For this review, take the finished solid that the model builds, in its own axes (mm). Round coordinates to 2 decimals unless told otherwise and drop trailing zeros. Answer in a Markdown table with one row per item. Add a question column.
from build123d import *

# Parameters (mm, degrees)
SKETCH1_W           = 52
SKETCH1_H           = 18
BOSS_EXTRUDE1_DEPTH = 6.55
FILLET1_R           = 2
FILLET2_R           = 1
SKETCH2_W           = 45
SKETCH2_H           = 14
CUT_EXTRUDE1_DEPTH  = 0.01
SKETCH3_W           = 14
SKETCH3_H           = 8
CUT_EXTRUDE2_DEPTH  = 0.01


with BuildPart() as part:
    # Sketch1 → Boss-Extrude1 (new, symmetric)
    with BuildSketch(Plane(origin=(0, 0, 0), x_dir=(1, 0, 0), z_dir=(0, 1, 0))):
        Rectangle(SKETCH1_W, SKETCH1_H)
    extrude(amount=BOSS_EXTRUDE1_DEPTH, both=True)

    # Fillet1
    fillet1_edges = [part.edges().sort_by_distance(p)[0] for p in [
        (-26, 6.55, 0),
        (26, 6.55, 0),
        (-26, -6.55, 0),
        (26, -6.55, 0),
    ]]
    fillet(fillet1_edges, radius=FILLET1_R)

    # Fillet2
    fillet2_edges = [part.edges().sort_by_distance(p)[0] for p in [
        (-26, 0, 9),
        (-26, 0, -9),
        (0, -6.55, 9),
        (26, 0, 9),
        (0, 6.55, 9),
        (25.414213562, 5.964213562, 9),
        (25.414213562, -5.964213562, 9),
        (-25.414213562, 5.964213562, 9),
        (-25.414213562, -5.964213562, 9),
        (0, -6.55, -9),
        (0, 6.55, -9),
        (26, 0, -9),
        (25.414213562, 5.964213562, -9),
        (25.414213562, -5.964213562, -9),
        (-25.414213562, 5.964213562, -9),
        (-25.414213562, -5.964213562, -9),
    ]]
    fillet(fillet2_edges, radius=FILLET2_R)

    # Sketch2 → Cut-Extrude1 (cut)
    with BuildSketch(Plane(origin=(0, 6.55, 0), x_dir=(1, 0, 0), z_dir=(0, 1, 0))):
        Rectangle(SKETCH2_W, SKETCH2_H)
    cut_extrude1 = extrude(amount=-CUT_EXTRUDE1_DEPTH, mode=Mode.SUBTRACT)

    # Sketch3 → Cut-Extrude2 (cut)
    with BuildSketch(Plane.ZY.offset(26)):
        Rectangle(SKETCH3_W, SKETCH3_H)
    cut_extrude2 = extrude(amount=-CUT_EXTRUDE2_DEPTH, mode=Mode.SUBTRACT)

    # Mirror3: Cut-Extrude1 across plane
    add(cut_extrude1.mirror(Plane.ZX), mode=Mode.SUBTRACT)

    # Mirror4: Cut-Extrude2 across plane
    add(cut_extrude2.mirror(Plane(origin=(0, 0, 0), x_dir=(0, 0, 1), z_dir=(1, 0, 0))), mode=Mode.SUBTRACT)


solid = part.part
Q1. Insertion check: pin 1 Ø1 at (x, z) = (13, 2) entering from -Y; pin 2 Ø3 at (y, z) = (-1, -3.5) entering from -X; pin 3 Ø1.5 at (x, z) = (-20.5, 2.5) entering from +Y. Each pin has a flat end and moves straight along its axis. Give the tip position at first contact, or say it passes through.
Q2. Draft analysis for pull direction Y (two halves, no side actions). For faces 1 (the face through (-25.43, 5.95, -0.11)), 2 (the face through (-0.1, -6.55, 7.7)), 3 (the face through (-26, -4.4, 0)), state which applies: released by +Y, released by -Y, zero draft, split by the parting line, or undercut.
Q3. To check wall thickness, follow probe 1 along X at (y, z) = (-4.75, 8); probe 2 along Y at (x, z) = (-22, -0.5); probe 3 along Y at (x, z) = (-18.5, -8.5). State the ranges of each line that lie inside material, in increasing order.
Answer sheet:
| question | item | result |
|---|---|---|
| 1 | pin 1 | stops at y = -6.54 |
| 1 | pin 2 | stops at x = -25.99 |
| 1 | pin 3 | stops at y = 6.54 |
| 2 | face 1 | released by +Y |
| 2 | face 2 | released by -Y |
| 2 | face 3 | zero draft |
| 3 | probe 1 | x = -25.99 to 25.99 |
| 3 | probe 2 | y = -6.54 to 6.54 |
| 3 | probe 3 | y = -6.42 to 6.42 |
